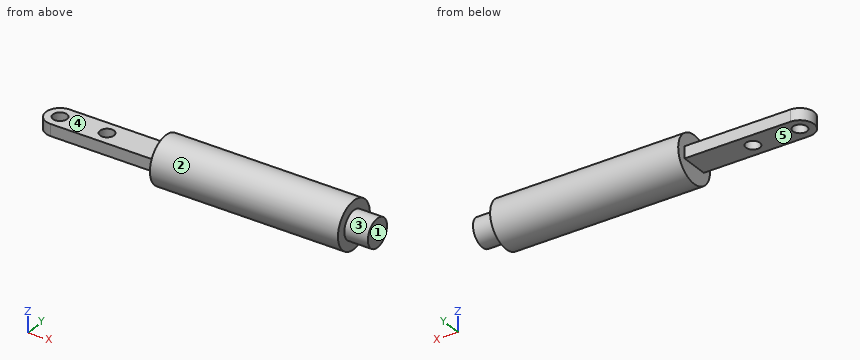
from build123d import *

# Parameters (mm, degrees)
SKETCH2_R           = 3
BOSS_EXTRUDE1_DEPTH = 2.5


with BuildPart() as part:
    # Sketch1 → Revolve1 (revolve)
    with BuildSketch(Plane(origin=(0, 0, 0), x_dir=(1, 0, 0), z_dir=(0, 1, 0)), mode=Mode.PRIVATE) as revolve1_sk:
        Polygon((80, 10), (0, 10), (0, 0), (90, 0), (90, 6), (80, 6), align=None)
    revolve(revolve1_sk.sketch.rotate(Axis((0, 0, 0), (1, 0, 0)), 180), axis=Axis((0, 0, 0), (1, 0, 0)))

    # Sketch2 → Boss-Extrude1 (add, symmetric)
    with BuildSketch(Plane.XY):
        with BuildLine():
            Line((0, -6), (0, 6))
            Line((0, 6), (-45, 6))
            ThreePointArc((-45, 6), (-51, 0), (-45, -6))
            Line((-45, -6), (0, -6))
        make_face()
        with Locations((-25, 0)):
            Circle(SKETCH2_R, mode=Mode.SUBTRACT)
        with Locations((-45, 0)):
            Circle(SKETCH2_R, mode=Mode.SUBTRACT)
    extrude(amount=BOSS_EXTRUDE1_DEPTH, both=True)


solid = part.part
Design review of the part built by this model. Coordinates are the model's own, in mm. Face numbers are marked on the shaded views. A direction names the side the tool comes from. Round coordinates to 2 decimals unless told otherwise and drop trailing zeros. Loops run counter-clockwise (first coordinate to the right, second up) from the corner with the lowest first, then second, coordinate; pieces in that order, holes last. Notation, with made-up numbers: M 85,-5 L 141,-5 A20 cw 141,-1 Z; hole C -40,89.5 d4. An arc over 180 degrees is marked long. Answer as a JSON object with one key per item and string values.
Item 1: Clearance check with flat-ended pins moving along their axes: P1, Ø6, axis at x = 25, z = 4, coming from the +Y side; P2, Ø4, axis at x = -30, z = -0.5, coming from the +Y side; P3, Ø6, axis at x = -13, y = 3, coming from the -Z side; P4, Ø3.5, axis at x = -25, y = 0, coming from the -Z side. State where each tip first meets the part, or that it passes through.
Answer sheet:
{"P1": "stops at y = 9.95", "P2": "stops at y = 6", "P3": "stops at z = -2.5", "P4": "passes through"}
Item 2: Wall thickness on L1, parallel to Y at x = -45, z = -0.9; L2, parallel to Y at x = 40, z = -0.5; L3, parallel to X at y = -0.25, z = 4.25: over which ranges is each line inside the solid? List them lowest first. Write a range as from..to.
Answer sheet:
{"L1": "y = -6..-3, 3..6", "L2": "y = -9.99..9.99", "L3": "x = 0..90"}
Item 3: Machinability: for the marked faces 1, 2, 3, 4 and 5, which of the approach directions +Z, -Z, +X, -X, +Y, -Y give a long, thin tool a straight path to every point of the face, cutting with its end or side? Answer none if there is none.
Answer sheet:
{"face 1": "+Z, -Z, +X, +Y, -Y", "face 2": "+X, -X", "face 3": "+X", "face 4": "+Z, -X, +Y, -Y", "face 5": "-Z, -X, +Y, -Y"}
Item 4: We need section C-C on z = -3.75. Give the boundary of the cut face in (x, y).
Answer sheet:
{"outline": "M 0,-9.27 L 80,-9.27 L 80,-4.68 L 90,-4.68 L 90,4.68 L 80,4.68 L 80,9.27 L 0,9.27 Z"}
Item 5: We need section B-B on x = -25. Give the boundary of the cut face in (y, z).
Answer sheet:
{"outline": "M -6,-2.5 L -3,-2.5 L -3,2.5 L -6,2.5 Z; M 3,-2.5 L 6,-2.5 L 6,2.5 L 3,2.5 Z"}
Item 6: We need section A-A on y = 0. Give the boundary of the cut face in (x, z).
Answer sheet:
{"outline": "M -51,-2.5 L -48,-2.5 L -48,2.5 L -51,2.5 Z; M -42,-2.5 L -28,-2.5 L -28,2.5 L -42,2.5 Z; M -22,-2.5 L 0,-2.5 L 0,-10 L 80,-10 L 80,-6 L 90,-6 L 90,6 L 80,6 L 80,10 L 0,10 L 0,2.5 L -22,2.5 Z"}
Item 7: We need section D-D on x = 56. Give the boundary of the cut face in (y, z), and give its area (3 significant figures).
Answer sheet:
{"outline": "C 0,0 d20", "area": "314 mm^2"}
